Study the drawing (mm; zero at the part's minimum x, y, z) and answer. A direction names the side the tool comes from. Give positions to 0.01 mm unless a question says otherwise; leave off trailing zeros. Write each loop counter-clockwise with the first axis right and the second up, starting at its lowest first coordinate (ties: lowest second). Pieces come first, ordered by that corner, then holes. Notation, with made-up numbers: (34.5, 35) - (79.5, 35) arc R16 ccw to (79.5, 55) - close; hole circle Ø4 at (9.5, -8). An arc over 180 degrees is marked (long way). Return JSON: item names as keys, results as strings.
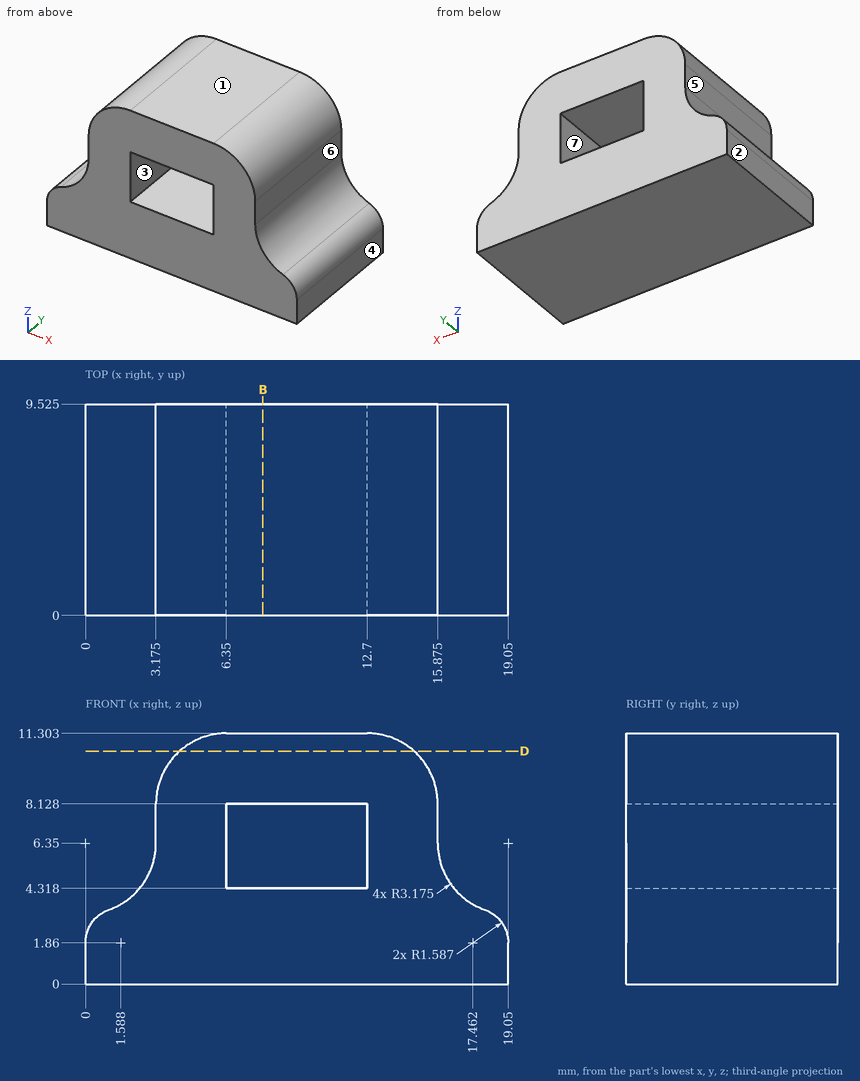
Item 1: Flat-ended cylindrical pins translate along their axes: P1, Ø1.9, axis at y = 3, z = 7, coming from the +X side; P2, Ø4, axis at y = 4.5, z = 5.5, coming from the -X side; P3, Ø3, axis at y = 7, z = 5.5, coming from the -X side (1 decimal). Find the tip coordinate at first contact, or state that the pin passes through.
Answer below:
{"P1": "stops at x = 15.89", "P2": "stops at x = 1.4", "P3": "stops at x = 2.1"}
Item 2: The mould has two halves that part along X. Classify the marked faces 1, 2, 3 and 4: +X half, -X half, draft (parallel to the pull), parting line (faces both ways), or undercut.
Answer below:
{"face 1": "draft", "face 2": "-X half", "face 3": "undercut", "face 4": "+X half"}
Item 3: Consider L1, parallel to Z at x = 11, y = 5.5; L2, parallel to Z at x = 18, y = 1 (1 decimal); L3, parallel to X at y = 3.25, z = 5.5. Determine where each line is inside the solid, lowest interval first.
Answer below:
{"L1": "z = 0 to 4.32, 8.13 to 11.3", "L2": "z = 0 to 3.4", "L3": "x = 3.06 to 6.35, 12.7 to 15.99"}
Item 4: For the marked faces 5, 6 and 7, determine the directions among +Z, -Z, +X, -X, +Y, -Y from which every point of the face is accessible in a straight line to the end or side of a thin tool.
Answer below:
{"face 5": "+Z, -X, +Y, -Y", "face 6": "+Z, +X, +Y, -Y", "face 7": "+Y, -Y"}
Item 5: A cutting plane is placed at D-D on z = 10.5. Determine the outline of the cut face in (x, y) (1 decimal).
Answer below:
{"outline": "(4.2, 0) - (14.8, 0) - (14.8, 9.5) - (4.2, 9.5) - close"}
Item 6: A cutting plane is placed at B-B on x = 8. Determine the outline of the cut face in (y, z) (1 decimal).
Answer below:
{"outline": "(0, 0) - (9.5, 0) - (9.5, 4.3) - (0, 4.3) - close; (0, 8.1) - (9.5, 8.1) - (9.5, 11.3) - (0, 11.3) - close"}
